from build123d import *

# Parameters (mm, degrees)
SKETCH1_W               = 45.8
SKETCH1_H               = 36.6
BOSS_EXTRUDE1_DEPTH     = 2
SKETCH2_R               = 13
BOSS_EXTRUDE2_DEPTH     = 13.84
SKETCH5_W               = 9
SKETCH5_H               = 16
BOSS_EXTRUDE3_DEPTH     = 13.84249374
CUT_EXTRUDE2_REACH      = 36.016
CUT_EXTRUDE2_END_RADIUS = 13
SKETCH7_R               = 2.85
CUT_EXTRUDE3_DEPTH      = 1.75
CUT_EXTRUDE3_DEPTH_BACK = 1.75
SKETCH9_W               = 7.5
SKETCH9_H               = 13.84


with BuildPart() as part:
    # Sketch1 → Boss-Extrude1 (new body)
    with BuildSketch(Plane(origin=(0, 0, 0), x_dir=(1, 0, 0), z_dir=(0, 1, 0))):
        with Locations((-1, 0)):
            Rectangle(SKETCH1_W, SKETCH1_H)
    extrude(amount=BOSS_EXTRUDE1_DEPTH)

    # Sketch2 → Boss-Extrude2 (add)
    with BuildSketch(Plane(origin=(0, 2, 0), x_dir=(1, 0, 0), z_dir=(0, 1, 0))):
        with Locations(Location((0, 0, 0), (0, 0, 270))):
            Circle(SKETCH2_R)
    extrude(amount=BOSS_EXTRUDE2_DEPTH)

    # Sketch5 → Boss-Extrude3 (add)
    with BuildSketch(Plane(origin=(0, 2, 0), x_dir=(1, 0, 0), z_dir=(0, 1, 0))):
        with Locations((12.5, 0)):
            Rectangle(SKETCH5_W, SKETCH5_H)
    extrude(amount=BOSS_EXTRUDE3_DEPTH)

    # Sketch6 → Cut-Revolve1 (revolve, cut)
    with BuildSketch(Plane.XY):
        with BuildLine():
            Line((0, 19.5), (0, 3.2))
            ThreePointArc((0, 3.2), (8.15, 11.35), (0, 19.5))
        make_face()
    revolve(axis=Axis((0, 3.2, 0), (0, 1, 0)), mode=Mode.SUBTRACT)

    # Cut-Extrude2: up to this cylinder (the profile starts inside it)
    cut_extrude2_end = Plane(origin=(0, 7.2, 0), z_dir=(0, -1, 0)) * Cylinder(CUT_EXTRUDE2_END_RADIUS, 99.032, mode=Mode.PRIVATE)
    # Sketch7 → Cut-Extrude2 (cut, up to the surface)
    with BuildSketch(Plane.XY, mode=Mode.PRIVATE) as cut_extrude2_sk1:
        with Locations((0, 7.2)):
            Circle(SKETCH7_R)
    cut_extrude2_tool1 = extrude(cut_extrude2_sk1.sketch, amount=-CUT_EXTRUDE2_REACH, mode=Mode.PRIVATE) & cut_extrude2_end
    add(cut_extrude2_tool1.solids().sort_by_distance((0, 7.2, 0))[0], mode=Mode.SUBTRACT)

    # Sketch9 → Cut-Extrude3 (cut, two sides: drawn at the far end of the back side and taken through both)
    with BuildSketch(Plane.XY.offset(-CUT_EXTRUDE3_DEPTH_BACK)):
        with Locations((-9.25, 8.92)):
            Rectangle(SKETCH9_W, SKETCH9_H)
    extrude(amount=CUT_EXTRUDE3_DEPTH + CUT_EXTRUDE3_DEPTH_BACK, mode=Mode.SUBTRACT)


solid = part.part
For this review, take the finished solid that the model builds, in its own axes (mm). A direction names the side the tool comes from. Round coordinates to 2 decimals unless told otherwise and drop trailing zeros. Loops run counter-clockwise (first coordinate to the right, second up) from the corner with the lowest first, then second, coordinate; pieces in that order, holes last. Notation, with made-up numbers: (-0.75, -38.75) - (22.25, -38.75) arc R24 cw to (22.25, -12.75) - close; hole circle Ø4 at (43.25, 55.25). An arc over 180 degrees is marked (long way). One line per item, written item: value. Start each with the question number.
Item 1: Take a section at B-B (x = 1). Give the boundary of the cut face in (y, z), plus the area to 3 significant figures.
Item 2: Take a section at D-D (x = 13). Give the boundary of the cut face in (y, z).
Item 3: Take a section at A-A (z = 12). Give the boundary of the cut face in (x, y), plus the area to 3 significant figures.
Item 4: Clearance check with flat-ended pins moving along their axes: pin 1 Ø8 at (x, y) = (17, 10) entering from +Z; pin 2 Ø1.8 at (y, z) = (4, -0.5) entering from -X; pin 3 Ø3.5 at (x, y) = (-9.5, 12) entering from +Z. State where each tip first meets the part, or that it passes through.
Item 5: The part is to be moulded in two halves that separate along Y. For faces 5 (the flat face through (12, 15.842, 0)), 6 (the flat face through (13, 9, -8)), 7 (the cylindrical face through (-0.62, 4.42, -9.51)), 8 (the flat face through (-1, 0, 0)), say which applies: +Y half, -Y half, draft (parallel to the pull), parting line (faces both ways), or undercut.
Item 6: For L1, parallel to Y at x = 0, z = -8.25; L2, parallel to Z at x = 13, y = 2.25; L3, parallel to Y at x = -9.5, z = 12.5, list the stretches that pass through material, from the lowest coordinate up.
Item 7: Take a section at C-C (y = 9). Give the boundary of the cut face in (x, z), plus the area to 3 significant figures.
Item 8: For faces 1 (the cylindrical face through (-3.6, 8.82, 12.49)), 2 (the cylindrical face through (-3.2, 8.8, -12.6)), 3 (the flat face through (17, 9, 0)), 4 (the flat face through (-5.5, 4, 0)), list the 3-axis set-ups (+Z, -Z, +X, -X, +Y, -Y) from which the entire face can be reached by the end or side of a thin tool; tool diameter is ignored.
Answer below:
1. outline: (0, -18.3) - (2, -18.3) - (2, -12.96) - (4.53, -12.96) - (4.53, -4.35) arc R8.09 cw to (15.84, 6.73) - (15.84, 12.96) - (2, 12.96) - (2, 18.3) - (0, 18.3) - close; (9.87, -12.96) - (15.84, -12.96) - (15.84, -6.73) arc R8.09 cw to (9.87, -7.95) - close
1. area: 227 mm2
2. outline: (0, -18.3) - (2, -18.3) - (2, -8) - (15.84, -8) - (15.84, 8) - (2, 8) - (2, 18.3) - (0, 18.3) - close
3. outline: (-23.9, 0) - (21.9, 0) - (21.9, 2) - (5, 2) - (5, 15.84) - (-5, 15.84) - (-5, 2) - (-23.9, 2) - close
3. area: 230 mm2
4. pin 1: stops at z = 8
4. pin 2: stops at x = -5.5
4. pin 3: stops at z = 10.44
5. face 5: +Y half
5. face 6: draft
5. face 7: undercut
5. face 8: -Y half
6. L1: y = 0 to 4.35, 10.05 to 15.84
6. L2: z = -8 to 8
6. L3: y = 0 to 2
7. outline: (-12.88, -1.75) arc R13 ccw to (-2.21, -12.81) - (-2.21, -7.48) arc R7.8 cw to (-7.61, -1.75) - close; (-12.88, 1.75) - (-7.61, 1.75) arc R7.8 cw (long way) to (2.21, -7.48) - (2.21, -12.81) arc R13 ccw to (10.25, -8) - (17, -8) - (17, 8) - (10.25, 8) arc R13 ccw to start
7. area: 376 mm2
8. face 1: +Z, +Y
8. face 2: -Z, +Y
8. face 3: +Z, -Z, +X, +Y
8. face 4: -X, +Y
